from build123d import *

# Parameters (mm, degrees)
SKETCH1_W           = 304.8
SKETCH1_H           = 316.8
BOSS_EXTRUDE1_DEPTH = 6
SKETCH3_W           = 42
SKETCH3_H           = 43.653543308
CUT_EXTRUDE2_DEPTH  = 220.891609663
SKETCH4_R           = 1.5
CUT_EXTRUDE3_DEPTH  = 220.891609663
SKETCH5_R           = 3.175
CUT_EXTRUDE4_DEPTH  = 220.891609663


with BuildPart() as part:
    # Sketch1 → Boss-Extrude1 (new body)
    with BuildSketch(Plane.XY):
        Rectangle(SKETCH1_W, SKETCH1_H)
    extrude(amount=BOSS_EXTRUDE1_DEPTH)

    # Sketch3 → Cut-Extrude2 (cut, through all)
    with BuildSketch(Plane.XY.offset(6)):
        with Locations((-76.2, 79.2)):
            Rectangle(SKETCH3_W, SKETCH3_H)
        with Locations((76.2, 79.2)):
            Rectangle(SKETCH3_W, SKETCH3_H)
        with Locations((76.2, -79.2)):
            Rectangle(SKETCH3_W, SKETCH3_H)
        with Locations((-76.2, -79.2)):
            Rectangle(SKETCH3_W, SKETCH3_H)
    extrude(amount=-CUT_EXTRUDE2_DEPTH, mode=Mode.SUBTRACT)

    # Sketch4 → Cut-Extrude3 (cut, through all)
    with BuildSketch(Plane.XY.offset(6)):
        Circle(SKETCH4_R)
    extrude(amount=-CUT_EXTRUDE3_DEPTH, mode=Mode.SUBTRACT)

    # Sketch5 → Cut-Extrude4 (cut, through all)
    with BuildSketch(Plane.XY.offset(6)):
        with Locations((20, 0)):
            Circle(SKETCH5_R)
    extrude(amount=-CUT_EXTRUDE4_DEPTH, mode=Mode.SUBTRACT)


solid = part.part
For this review, take the finished solid that the model builds, in its own axes (mm). Give positions to 0.01 mm unless a question says otherwise; leave off trailing zeros. Loops run counter-clockwise (first coordinate to the right, second up) from the corner with the lowest first, then second, coordinate; pieces in that order, holes last. Notation, with made-up numbers: M 39.25,-1.75 L 92.25,-1.75 A7 cw 92.25,9.25 Z; hole C 89.5,45 d5. An arc over 180 degrees is marked long. Answer as a JSON object with one key per item and string values. Group by question number.
Q1. Insertion check: P1, Ø2, axis at x = 40, y = -49, coming from the -Z side. The pin has a flat end and moves straight along its axis. Give the tip position at first contact, or say it passes through.
Q2. For probe 1 along Y at (x, z) = (-89.5, 4.25); probe 2 along X at (y, z) = (-82, 2.75); probe 3 along Y at (x, z) = (20, 2.2) (3 decimals), list the stretches that pass through material, from the lowest coordinate up. Write a range as [from, to].
Q3. Add section C-C on x = -77. Give the boundary of the cut face in (y, z), and give its area (3 significant figures).
Q4. Add section B-B on z = 3.5. Give the boundary of the cut face in (x, y) (3 decimals).
Q5. Add section A-A on y = 62. Give the boundary of the cut face in (x, z), and give its area (3 significant figures).
Checked values:
{
 "1": {"P1": "z = 0"},
 "2": {"probe 1": "[-158.4, -101.03], [-57.37, 57.37], [101.03, 158.4]", "probe 2": "[-152.4, -97.2], [-55.2, 55.2], [97.2, 152.4]", "probe 3": "[-158.4, -3.175], [3.175, 158.4]"},
 "3": {"outline": "M -158.4,0 L -101.03,0 L -101.03,6 L -158.4,6 Z; M -57.37,0 L 57.37,0 L 57.37,6 L -57.37,6 Z; M 101.03,0 L 158.4,0 L 158.4,6 L 101.03,6 Z", "area": "1,380 mm²"},
 "4": {"outline": "M -152.4,-158.4 L 152.4,-158.4 L 152.4,158.4 L -152.4,158.4 Z; hole M -97.2,-101.027 L -55.2,-101.027 L -55.2,-57.373 L -97.2,-57.373 Z; hole M -97.2,57.373 L -55.2,57.373 L -55.2,101.027 L -97.2,101.027 Z; hole C 0,0 d3; hole C 20,0 d6.35; hole M 55.2,-101.027 L 97.2,-101.027 L 97.2,-57.373 L 55.2,-57.373 Z; hole M 55.2,57.373 L 97.2,57.373 L 97.2,101.027 L 55.2,101.027 Z"},
 "5": {"outline": "M -152.4,0 L -97.2,0 L -97.2,6 L -152.4,6 Z; M -55.2,0 L 55.2,0 L 55.2,6 L -55.2,6 Z; M 97.2,0 L 152.4,0 L 152.4,6 L 97.2,6 Z", "area": "1,320 mm²"}
}
